Source: CAD feature listing. Evaluate the final solid. Frame: model axes, mm. Give positions to 0.01 mm unless a question says otherwise; leave off trailing zeros. Order: outer loops, then holes, each group sorted by start corner. A loop starts at its lowest first (then second) coordinate and runs counter-clockwise, first axis right, second up.
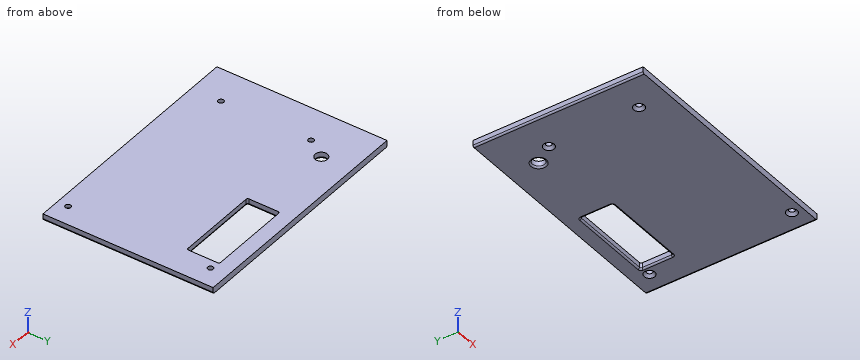
```python
from build123d import *

# Parameters (mm, degrees)
SKETCH1_W                     = 150
SKETCH1_H                     = 105
BOSS_EXTRUDE1_DEPTH           = 2
M3_CLEARANCE_HOLE1_AT_2_COUNT = 2
M3_CLEARANCE_HOLE1_AT_2_PITCH = 55.63
M3_CLEARANCE_HOLE1_AT_3_COUNT = 2
M3_CLEARANCE_HOLE1_AT_3_PITCH = 133.742517548
M3_CLEARANCE_HOLE1_AT_4_COUNT = 2
M3_CLEARANCE_HOLE1_AT_4_PITCH = 117.386327142
M7_CLEARANCE_HOLE1_D          = 7.6
SKETCH6_W                     = 52.2
SKETCH6_H                     = 20.1
CUT_EXTRUDE1_DEPTH            = 10
FILLET1_R                     = 1
FILLET2_R                     = 1
FILLET3_R                     = 1


with BuildPart() as part:
    # Sketch1 → Boss-Extrude1 (new, symmetric)
    with BuildSketch(Plane.XY):
        Rectangle(SKETCH1_W, SKETCH1_H)
    extrude(amount=BOSS_EXTRUDE1_DEPTH, both=True)

    # Sketch3 → M3 Clearance Hole1 (revolve, cut)
    with BuildSketch(Plane(origin=(-53, 21.4, 2), x_dir=(0, -1, 0), z_dir=(1, 0, 0))):
        Polygon((0, 0), (0, 4), (3.3, 4), (1.7, 2.4), (1.7, 0), align=None)
    m3_clearance_hole1 = revolve(axis=Axis((-53, 21.4, 8.35), (0, 0, -1)), mode=Mode.SUBTRACT)

    # M3 Clearance Hole1 at 2: M3 Clearance Hole1 ×2
    with Locations(*[(0, -i * M3_CLEARANCE_HOLE1_AT_2_PITCH, 0) for i in range(1, M3_CLEARANCE_HOLE1_AT_2_COUNT)]):
        add(m3_clearance_hole1, mode=Mode.SUBTRACT)

    # M3 Clearance Hole1 at 3: M3 Clearance Hole1 ×2
    with Locations(*[Vector(0.8641231084854607, -0.5032804917552683, 0) * (i * M3_CLEARANCE_HOLE1_AT_3_PITCH) for i in range(1, M3_CLEARANCE_HOLE1_AT_3_COUNT)]):
        add(m3_clearance_hole1, mode=Mode.SUBTRACT)

    # M3 Clearance Hole1 at 4: M3 Clearance Hole1 ×2
    with Locations(*[Vector(0.9845269275673837, 0.17523335554262423, 0) * (i * M3_CLEARANCE_HOLE1_AT_4_PITCH) for i in range(1, M3_CLEARANCE_HOLE1_AT_4_COUNT)]):
        add(m3_clearance_hole1, mode=Mode.SUBTRACT)

    # M7 Clearance Hole1 (through all)
    with Locations(Plane.XY.offset(2)):
        with Locations((-44.87, 33.54)):
            Hole(M7_CLEARANCE_HOLE1_D / 2)

    # Sketch6 → Cut-Extrude1 (cut)
    with BuildSketch(Plane.XY.offset(2)):
        with Locations((30.82, 33.37)):
            Rectangle(SKETCH6_W, SKETCH6_H)
    extrude(amount=-CUT_EXTRUDE1_DEPTH, mode=Mode.SUBTRACT)

    # Fillet1
    fillet1_edges = [part.edges().sort_by_distance(p)[0] for p in [
        (56.92, 33.37, -2),
        (30.82, 43.42, -2),
        (4.72, 33.37, -2),
        (30.82, 23.32, -2),
        (56.92, 23.32, 0),
        (4.72, 23.32, 0),
        (4.72, 43.42, 0),
        (56.92, 43.42, 0),
    ]]
    fillet(fillet1_edges, radius=FILLET1_R)

    # Fillet2
    fillet2_edges = [part.edges().sort_by_distance(p)[0] for p in [
        (-41.07, 33.54, -2),
    ]]
    fillet(fillet2_edges, radius=FILLET2_R)

    # Fillet3
    fillet3_edges = [part.edges().sort_by_distance(p)[0] for p in [
        (75, 0, -2),
        (-75, 0, -2),
    ]]
    fillet(fillet3_edges, radius=FILLET3_R)


solid = part.part
```
1) Section query A-A, the plane y = 33.54. Return the cut outline in (x, z), and give its area (3 significant figures).
Report:
outline: (-75, -1) arc R1 ccw to (-74, -2) - (-49.67, -2) arc R1 ccw to (-48.67, -1) - (-48.67, 2) - (-75, 2) - close; (-41.07, -1) arc R1 ccw to (-40.07, -2) - (3.72, -2) arc R1 ccw to (4.72, -1) - (4.72, 2) - (-41.07, 2) - close; (56.92, -1) arc R1 ccw to (57.92, -2) - (74, -2) arc R1 ccw to (75, -1) - (75, 2) - (56.92, 2) - close
area: 360 mm2
2) Pin query (flat end, axial travel): pin 1 (2 mm diameter, centred on x = 62.57, y = -45.91, fed in from +Z); pin 2 (4.5 mm diameter, centred on x = -53, y = -34.23, fed in from -Z); pin 3 (4.5 mm diameter, centred on x = 62.57, y = 41.97, fed in from +Z); pin 4 (5.5 mm diameter, centred on x = -53, y = 21.4, fed in from -Z). Return the tip coordinate at first contact, or that it passes through.
Report:
pin 1: passes through
pin 2: stops at z = -0.95
pin 3: stops at z = 2
pin 4: stops at z = -1.45
3) Material intervals for L1, parallel to Y at x = -53, z = 0.4; L2, parallel to X at y = -45.91, z = 1.4; L3, parallel to Y at x = -44.87, z = -0.1, sorted ascending.
Report:
L1: y = -52.5 to -35.93, -32.53 to 19.7, 23.1 to 52.5
L2: x = -75 to 60.87, 64.27 to 75
L3: y = -52.5 to 29.74, 37.34 to 52.5
4) Section query B-B, the plane x = -44.87. Return the cut outline in (y, z), and give its area (3 significant figures).
Report:
outline: (-52.5, -2) - (28.74, -2) arc R1 ccw to (29.74, -1) - (29.74, 2) - (-52.5, 2) - close; (37.34, -1) arc R1 ccw to (38.34, -2) - (52.5, -2) - (52.5, 2) - (37.34, 2) - close
area: 389 mm2
5) Section query D-D, the plane z = 1.15. Return the cut outline in (x, y).
Report:
outline: (-75, -52.5) - (75, -52.5) - (75, 52.5) - (-75, 52.5) - close; hole circle Ø3.4 at (-53, -34.23); hole circle Ø3.4 at (-53, 21.4); hole circle Ø7.6 at (-44.87, 33.54); hole (4.72, 24.32) arc R1 ccw to (5.72, 23.32) - (55.92, 23.32) arc R1 ccw to (56.92, 24.32) - (56.92, 42.42) arc R1 ccw to (55.92, 43.42) - (5.72, 43.42) arc R1 ccw to (4.72, 42.42) - close; hole circle Ø3.4 at (62.57, -45.91); hole circle Ø3.4 at (62.57, 41.97)
6) Section query C-C, the plane y = -34.23. Return the cut outline in (x, z).
Report:
outline: (-75, -1) arc R1 ccw to (-74, -2) - (-56.3, -2) - (-54.7, -0.4) - (-54.7, 2) - (-75, 2) - close; (-51.3, -0.4) - (-49.7, -2) - (74, -2) arc R1 ccw to (75, -1) - (75, 2) - (-51.3, 2) - close
